The model under review builds one solid part; all positions refer to its coordinate system, in mm. Face numbers are marked on the shaded views. A direction names the side the tool comes from. Coordinates: 2 decimals unless noted, no trailing zeros. Write each loop counter-clockwise with the first axis right and the second up, starting at its lowest first coordinate (ties: lowest second). Pieces come first, ordered by that corner, then holes. Notation, with made-up numbers: (-29.75, 57.25) - (-18.75, 57.25) arc R8 cw to (-18.75, 66.25) - close; hole circle Ø4 at (88.5, 22.25). An arc over 180 degrees is marked (long way). Answer as CSV lines item,"result". Start each with the question number.
```python
from build123d import *

# Parameters (mm, degrees)
BOSS_EXTRUDE1_DEPTH = 10
FILLET1_R           = 0.5
SKETCH2_R           = 1.515
CUT_EXTRUDE1_DEPTH  = 127.166955858
FILLET2_R           = 0.5


with BuildPart() as part:
    # Sketch1 → Boss-Extrude1 (new body)
    with BuildSketch(Plane.XY):
        with BuildLine():
            Line((0, 0), (0, 80))
            ThreePointArc((0, 80), (-8.82808737, 80.510568582), (-5.446921008, 88.681463327))
            ThreePointArc((-5.446921008, 88.681463327), (-33.19088971, 105.018694036), (-65, 110))
            ThreePointArc((-65, 110), (-36.020401707, 94.064120743), (-23.327746863, 63.524541867))
            Line((-23.327746863, 63.524541867), (-18.907194485, 65.860931532))
            ThreePointArc((-18.907194485, 65.860931532), (-13.559533082, 64.289226454), (-10, 60))
            Line((-10, 60), (-10, 0))
            Line((-10, 0), (0, 0))
        make_face()
    extrude(amount=BOSS_EXTRUDE1_DEPTH)

    # Fillet1
    fillet1_edges = [part.edges().sort_by_distance(p)[0] for p in [
        (-10, 60, 5),
        (-23.327746863, 63.524541867, 5),
        (-65, 110, 5),
        (-5.446921008, 88.681463327, 5),
        (0, 80, 5),
    ]]
    fillet(fillet1_edges, radius=FILLET1_R)

    # Sketch2 → Cut-Extrude1 (cut, through all)
    with BuildSketch(Plane.XY.offset(10)):
        with Locations((-5, 5)):
            Circle(SKETCH2_R)
        with Locations((-5, 19)):
            Circle(SKETCH2_R)
    extrude(amount=-CUT_EXTRUDE1_DEPTH, mode=Mode.SUBTRACT)

    # Fillet2
    fillet2_edges = [part.edges().sort_by_distance(p)[0] for p in [
        (-10, 0, 5),
        (0, 0, 5),
    ]]
    fillet(fillet2_edges, radius=FILLET2_R)


solid = part.part
```
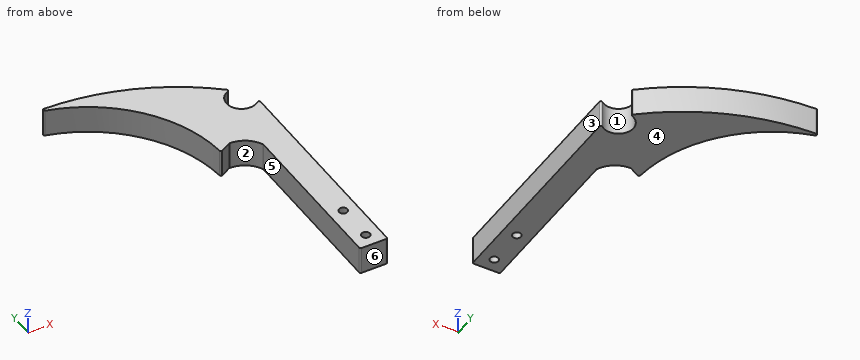
(1) Add section C-C on x = -52.5. Give the boundary of the cut face in (y, z), then the cut area to 3 significant figures.
(2) For pin 1 (10 mm diameter, centred on x = -4.23, y = 83.39, fed in from -Z); pin 2 (5 mm diameter, centred on y = 50, z = 2, fed in from -X); pin 3 (4 mm diameter, centred on x = -5, y = 19, fed in from -Z); pin 4 (1 mm diameter, centred on x = -20, z = 7, fed in from -Y), all flat-tipped, find the tip position at first contact; note any pin that passes through.
(3) Wall thickness on line 1 (Y direction, x = -5, z = 5.25) (3 decimals); line 2 (X direction, y = 45.5, z = 1.75); line 3 (X direction, y = 5.5, z = 7.75): over which ranges is each line inside the solid? List them lowest first.
(4) The part is to be moulded in two halves that separate along X. For the marked faces 1, 2, 3 and 4, say which applies: released by +X, released by -X, zero draft, split by the parting line, or undercut.
(5) Add section A-A on y = 19. Give the boundary of the cut face in (x, z) (3 decimals), then the cut area to 3 significant figures.
(6) Add section B-B on y = 56.5. Give the boundary of the cut face in (x, z).
(7) Add section D-D on z = 8.5. Give the number of separate pieces and of enclosed holes in the cut face, then the cut area to 3 significant figures.
(8) For the marked faces 5 and 6, list the 3-axis set-ups (+Z, -Z, +X, -X, +Y, -Y) from which the entire face can be reached by the end or side of a thin tool; tool diameter is ignored.
Reported:
1,outline,"(106.18, 0) - (109.5, 0) - (109.5, 10) - (106.18, 10) - close"
1,area,"33.3 mm²"
2,pin 1,"through"
2,pin 2,"x = -10"
2,pin 3,"z = 0"
2,pin 4,"y = 65.02"
3,line 1,"0 to 3.485, 6.515 to 17.485, 20.515 to 78.023"
3,line 2,"-10 to 0"
3,line 3,"-10 to -6.43, -3.57 to 0"
4,face 1,"undercut"
4,face 2,"undercut"
4,face 3,"released by +X"
4,face 4,"zero draft"
5,outline,"(-10, 0) - (-6.515, 0) - (-6.515, 10) - (-10, 10) - close; (-3.485, 0) - (0, 0) - (0, 10) - (-3.485, 10) - close"
5,area,"69.7 mm²"
6,outline,"(-10, 0) - (0, 0) - (0, 10) - (-10, 10) - close"
7,separate pieces,"1"
7,enclosed holes,"2"
7,area,"1,610 mm²"
8,face 5,"+Z, -Z, -X, -Y"
8,face 6,"+Z, -Z, +X, -X, -Y"
